from build123d import *

# Parameters (mm, degrees)
BOSS_EXTRUDE1_DEPTH = 3.175
CUT_EXTRUDE1_DEPTH  = 10
SKETCH3_R           = 2.0193
BOSS_EXTRUDE2_DEPTH = 3.175
FILLET1_R           = 10
FILLET2_R           = 50
SKETCH4_R           = 2.02
CUT_EXTRUDE2_DEPTH  = 10
SKETCH5_R           = 1.5
CUT_EXTRUDE3_DEPTH  = 10


with BuildPart() as part:
    # Sketch1 → Boss-Extrude1 (new body)
    with BuildSketch(Plane.XY):
        Polygon((165.934536959, -16.66935), (157.315236959, -8.05005), (115.359952094, -8.05005), (89.959952094, -8.05005), (48.004667228, -8.05005), (39.385367228, -16.66935), (39.385367228, -40.05005), (39.385367228, -52.41105), (165.934536959, -56.67505), (165.934536959, -42.05005), align=None)
        with BuildLine():
            ThreePointArc((47.685367228, -44.38075), (49.704667228, -46.40005), (47.685367228, -48.41935))
            ThreePointArc((47.685367228, -48.41935), (45.666067228, -46.40005), (47.685367228, -44.38075))
        make_face(mode=Mode.SUBTRACT)
        with BuildLine():
            ThreePointArc((47.685367228, -12.63075), (49.704667228, -14.65005), (47.685367228, -16.66935))
            ThreePointArc((47.685367228, -16.66935), (45.666067228, -14.65005), (47.685367228, -12.63075))
        make_face(mode=Mode.SUBTRACT)
        with BuildLine():
            ThreePointArc((73.085367228, -44.38075), (75.104667228, -46.40005), (73.085367228, -48.41935))
            ThreePointArc((73.085367228, -48.41935), (71.066067228, -46.40005), (73.085367228, -44.38075))
        make_face(mode=Mode.SUBTRACT)
        with BuildLine():
            ThreePointArc((73.085367228, -12.63075), (75.104667228, -14.65005), (73.085367228, -16.66935))
            ThreePointArc((73.085367228, -16.66935), (71.066067228, -14.65005), (73.085367228, -12.63075))
        make_face(mode=Mode.SUBTRACT)
        with BuildLine():
            ThreePointArc((132.234536959, -44.38075), (134.253836959, -46.40005), (132.234536959, -48.41935))
            ThreePointArc((132.234536959, -48.41935), (130.215236959, -46.40005), (132.234536959, -44.38075))
        make_face(mode=Mode.SUBTRACT)
        with BuildLine():
            ThreePointArc((132.234536959, -12.63075), (134.253836959, -14.65005), (132.234536959, -16.66935))
            ThreePointArc((132.234536959, -16.66935), (130.215236959, -14.65005), (132.234536959, -12.63075))
        make_face(mode=Mode.SUBTRACT)
        with BuildLine():
            ThreePointArc((157.634536959, -44.38075), (159.653836959, -46.40005), (157.634536959, -48.41935))
            ThreePointArc((157.634536959, -48.41935), (155.615236959, -46.40005), (157.634536959, -44.38075))
        make_face(mode=Mode.SUBTRACT)
        with BuildLine():
            ThreePointArc((157.634536959, -12.63075), (159.653836959, -14.65005), (157.634536959, -16.66935))
            ThreePointArc((157.634536959, -16.66935), (155.615236959, -14.65005), (157.634536959, -12.63075))
        make_face(mode=Mode.SUBTRACT)
        Polygon((115.359952094, -8.05005), (157.315236959, -8.05005), (115.359952094, 33.905234866), align=None)
        Polygon((89.959952094, -8.05005), (115.359952094, -8.05005), (115.359952094, 33.905234866), (115.359952094, 203.394265134), (115.359952094, 245.34955), (89.959952094, 245.34955), (89.959952094, 203.394265134), (89.959952094, 33.905234866), align=None)
        Polygon((48.004667228, -8.05005), (89.959952094, -8.05005), (89.959952094, 33.905234866), align=None)
        Polygon((89.959952094, 245.34955), (115.359952094, 245.34955), (157.315236959, 245.34955), (165.934536959, 253.96885), (165.934536959, 279.34955), (165.934536959, 293.97455), (39.385367228, 289.71055), (39.385367228, 277.34955), (39.385367228, 253.96885), (48.004667228, 245.34955), align=None)
        with BuildLine():
            ThreePointArc((47.685367228, 253.96885), (49.704667228, 251.94955), (47.685367228, 249.93025))
            ThreePointArc((47.685367228, 249.93025), (45.666067228, 251.94955), (47.685367228, 253.96885))
        make_face(mode=Mode.SUBTRACT)
        with BuildLine():
            ThreePointArc((47.685367228, 285.71885), (49.704667228, 283.69955), (47.685367228, 281.68025))
            ThreePointArc((47.685367228, 281.68025), (45.666067228, 283.69955), (47.685367228, 285.71885))
        make_face(mode=Mode.SUBTRACT)
        with BuildLine():
            ThreePointArc((73.085367228, 253.96885), (75.104667228, 251.94955), (73.085367228, 249.93025))
            ThreePointArc((73.085367228, 249.93025), (71.066067228, 251.94955), (73.085367228, 253.96885))
        make_face(mode=Mode.SUBTRACT)
        with BuildLine():
            ThreePointArc((73.085367228, 285.71885), (75.104667228, 283.69955), (73.085367228, 281.68025))
            ThreePointArc((73.085367228, 281.68025), (71.066067228, 283.69955), (73.085367228, 285.71885))
        make_face(mode=Mode.SUBTRACT)
        with BuildLine():
            ThreePointArc((132.234536959, 253.96885), (134.253836959, 251.94955), (132.234536959, 249.93025))
            ThreePointArc((132.234536959, 249.93025), (130.215236959, 251.94955), (132.234536959, 253.96885))
        make_face(mode=Mode.SUBTRACT)
        with BuildLine():
            ThreePointArc((157.634536959, 253.96885), (159.653836959, 251.94955), (157.634536959, 249.93025))
            ThreePointArc((157.634536959, 249.93025), (155.615236959, 251.94955), (157.634536959, 253.96885))
        make_face(mode=Mode.SUBTRACT)
        with BuildLine():
            ThreePointArc((157.634536959, 285.71885), (159.653836959, 283.69955), (157.634536959, 281.68025))
            ThreePointArc((157.634536959, 281.68025), (155.615236959, 283.69955), (157.634536959, 285.71885))
        make_face(mode=Mode.SUBTRACT)
        Polygon((115.359952094, 245.34955), (115.359952094, 203.394265134), (157.315236959, 245.34955), align=None)
        Polygon((48.004667228, 245.34955), (89.959952094, 203.394265134), (89.959952094, 245.34955), align=None)
    extrude(amount=BOSS_EXTRUDE1_DEPTH)

    # Sketch2 → Cut-Extrude1 (cut)
    with BuildSketch(Plane.XY.offset(3.175)):
        Polygon((84.385367228, -52.41105), (39.385367228, -52.41105), (165.934536959, -56.67505), (165.934536959, -52.41105), (120.934536959, -52.41105), align=None)
        Polygon((120.934536959, 289.71055), (165.934536959, 289.71055), (165.934536959, 293.97455), (39.385367228, 289.71055), (84.385367228, 289.71055), align=None)
    extrude(amount=-CUT_EXTRUDE1_DEPTH, mode=Mode.SUBTRACT)

    # Sketch3 → Boss-Extrude2 (add)
    with BuildSketch(Plane.XY.offset(3.175)):
        Polygon((37.385367228, -15.840922875), (37.385367228, -54.41105), (167.934536959, -54.41105), (167.934536959, -15.840922875), (117.359952094, 34.73366199), (117.359952094, 202.56583801), (167.934536959, 253.140422875), (167.934536959, 291.71055), (37.385367228, 291.71055), (37.385367228, 253.140422875), (87.959952094, 202.56583801), (87.959952094, 34.73366199), align=None)
        with Locations((132.234536959, -46.40005)):
            Circle(SKETCH3_R, mode=Mode.SUBTRACT)
        with Locations((132.234536959, -14.65005)):
            Circle(SKETCH3_R, mode=Mode.SUBTRACT)
        with Locations((47.685367228, -14.65005)):
            Circle(SKETCH3_R, mode=Mode.SUBTRACT)
        with Locations((47.685367228, -46.40005)):
            Circle(SKETCH3_R, mode=Mode.SUBTRACT)
        with Locations((73.085367228, -46.40005)):
            Circle(SKETCH3_R, mode=Mode.SUBTRACT)
        with Locations((73.085367228, -14.65005)):
            Circle(SKETCH3_R, mode=Mode.SUBTRACT)
        with Locations((157.634536959, -14.65005)):
            Circle(SKETCH3_R, mode=Mode.SUBTRACT)
        with Locations((157.634536959, -46.40005)):
            Circle(SKETCH3_R, mode=Mode.SUBTRACT)
        with Locations((132.234536959, 251.94955)):
            Circle(SKETCH3_R, mode=Mode.SUBTRACT)
        with Locations((73.085367228, 251.94955)):
            Circle(SKETCH3_R, mode=Mode.SUBTRACT)
        with Locations((157.634536959, 251.94955)):
            Circle(SKETCH3_R, mode=Mode.SUBTRACT)
        with Locations((47.685367228, 251.94955)):
            Circle(SKETCH3_R, mode=Mode.SUBTRACT)
        with Locations((47.685367228, 283.69955)):
            Circle(SKETCH3_R, mode=Mode.SUBTRACT)
        with Locations((73.085367228, 283.69955)):
            Circle(SKETCH3_R, mode=Mode.SUBTRACT)
        with Locations((157.634536959, 283.69955)):
            Circle(SKETCH3_R, mode=Mode.SUBTRACT)
    extrude(amount=-BOSS_EXTRUDE2_DEPTH)

    # Fillet1
    fillet1_edges = [part.edges().sort_by_distance(p)[0] for p in [
        (37.385367228, -54.41105, 1.5875),
        (167.934536959, -54.41105, 1.5875),
        (167.934536959, -15.840922875, 1.5875),
        (167.934536959, 253.140422875, 1.5875),
        (167.934536959, 291.71055, 1.5875),
        (37.385367228, 291.71055, 1.5875),
        (37.385367228, 253.140422875, 1.5875),
        (37.385367228, -15.840922875, 1.5875),
    ]]
    fillet(fillet1_edges, radius=FILLET1_R)

    # Fillet2
    fillet2_edges = [part.edges().sort_by_distance(p)[0] for p in [
        (117.359952094, 34.73366199, 1.5875),
        (117.359952094, 202.56583801, 1.5875),
        (87.959952094, 202.56583801, 1.5875),
        (87.959952094, 34.73366199, 1.5875),
    ]]
    fillet(fillet2_edges, radius=FILLET2_R)

    # Sketch4 → Cut-Extrude2 (cut)
    with BuildSketch(Plane.XY.offset(3.175)):
        with Locations((132.234536959, 283.69955)):
            Circle(SKETCH4_R)
    extrude(amount=-CUT_EXTRUDE2_DEPTH, mode=Mode.SUBTRACT)

    # Sketch5 → Cut-Extrude3 (cut)
    with BuildSketch(Plane(origin=(0, 0, 0), x_dir=(-1, 0, 0), z_dir=(0, 0, -1))):
        with Locations((-102.659952094, 58.64975)):
            Circle(SKETCH5_R)
        with Locations((-102.659952094, 98.64975)):
            Circle(SKETCH5_R)
        with Locations((-102.659952094, 138.64975)):
            Circle(SKETCH5_R)
        with Locations((-102.659952094, 178.64975)):
            Circle(SKETCH5_R)
        with Locations((-102.659952094, 18.64975)):
            Circle(SKETCH5_R)
        with Locations((-102.659952094, 218.64975)):
            Circle(SKETCH5_R)
    extrude(amount=-CUT_EXTRUDE3_DEPTH, mode=Mode.SUBTRACT)


solid = part.part
Could you check a few things on this model? Use its own coordinates, in mm. A direction names the side the tool comes from. Coordinates: 2 decimals unless noted, no trailing zeros. Write each loop counter-clockwise with the first axis right and the second up, starting at its lowest first coordinate (ties: lowest second). Pieces come first, ordered by that corner, then holes. Notation, with made-up numbers: M 35.5,-33 L 82.5,-33 A21 cw 82.5,-21 Z; hole C 72,15.5 d5. An arc over 180 degrees is marked long. One line per question, with ' | ' between items.
1) Imagine slicing it at C-C, the plane y = 131. Write out the boundary of the cut face in (x, z) (3 decimals).
Checks:
outline: M 87.96,0 L 117.36,0 L 117.36,3.175 L 87.96,3.175 Z
2) Imagine slicing it at B-B, the plane x = 124. Write out the boundary of the cut face in (y, z) (3 decimals).
Checks:
outline: M -54.411,0 L 30.546,0 L 30.546,3.175 L -54.411,3.175 Z; M 206.753,0 L 291.711,0 L 291.711,3.175 L 206.753,3.175 Z
3) Imagine slicing it at A-A, the plane x = 60. Write out the boundary of the cut face in (y, z) (3 decimals).
Checks:
outline: M -54.411,0 L 6.774,0 L 6.774,3.175 L -54.411,3.175 Z; M 230.526,0 L 291.711,0 L 291.711,3.175 L 230.526,3.175 Z
4) Imagine slicing it at D-D, the plane z = 2.2. Give the number of separate pieces and of enclosed holes in the cut face, and give its area (3 significant figures).
Checks:
separate pieces: 1 | enclosed holes: 22 | area: 23,000 mm²
5) I need wall thicknesses on probe 1 along Y at (x, z) = (133, 2.7); probe 2 along X at (y, z) = (183, 0.35); probe 3 along Y at (x, z) = (71, 1.35). Which ranges of each line are inside material? Lowest first, please. Write a range as [from, to].
Checks:
probe 1: [-54.41, -48.27], [-44.53, -16.52], [-12.78, 19.09], [218.21, 250.08], [253.82, 281.83], [285.57, 291.71] | probe 2: [87.95, 117.37] | probe 3: [-54.41, 17.77], [219.53, 291.71]
6) For faces 1 (the face through (165.083, -51.404, 1.565)), 2 (the face through (56.584, 233.942, 1.61)), 3 (the face through (148.274, 233.48, 1.61)), which set-ups out of +Z, -Z, +X, -X, +Y, -Y let a thin tool reach every point of the face, with its end or its side?
Checks:
face 1: +Z, -Z, +X, -Y | face 2: +Z, -Z, -X | face 3: +Z, -Z, +X
7) If we mould it in two halves opening along Y, with no side actions, what happens to faces 4 (the face through (121.27, 36.06, 1.57)), 5 (the face through (102, 121, 3.175)), 6 (the face through (164.927, 288.859, 1.565))? For each: released by +Y, released by -Y, zero draft, split by the parting line, or undercut.
Checks:
face 4: undercut | face 5: zero draft | face 6: released by +Y
8) For pin 1 Ø4.5 at (x, y) = (73.09, -46.4) entering from +Z (3 decimals); pin 2 Ø1.6 at (y, z) = (126, 1.5) entering from +X, each with a flat end and sliding along its axis, tell me the tip position at first contact or that it passes through.
Checks:
pin 1: z = 3.175 | pin 2: x = 117.36
